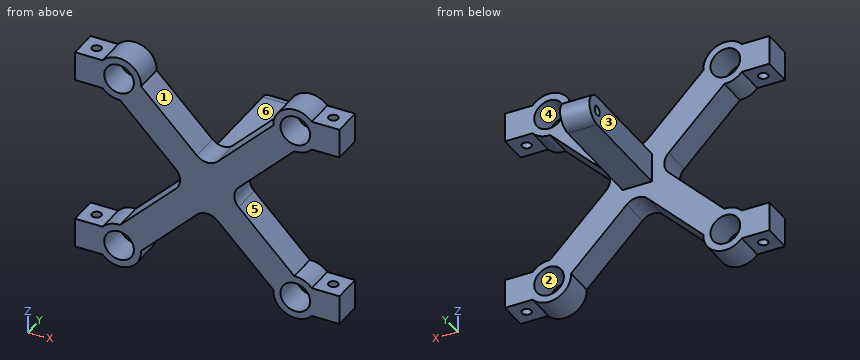
```python
from build123d import *

# Parameters (mm, degrees)
SKETCH_1_R          = 5.05
EXTRUDE_1_DEPTH     = 10
SKETCH_2_W          = 10
SKETCH_2_H          = 10
EXTRUDE_2_DEPTH     = 40
FILLET_3_RADIUS     = 5
FILLET_3_LENGTH     = 10
SKETCH_3_R          = 1.6
CUT_EXTRUDE_1_DEPTH = 81.039052968
SKETCH_4_R          = 1.6
CUT_EXTRUDE_2_DEPTH = 99.900202224


with BuildPart() as part:
    # ｽｹｯﾁ1 → ﾎﾞｽ - 押し出し1 (new body)
    with BuildSketch(Plane(origin=(0, 0, 0), x_dir=(1, 0, 0), z_dir=(0, 1, 0))):
        with BuildLine():
            Line((3.535533906, -10.677312396), (22.508173367, -29.649951857))
            ThreePointArc((22.508173367, -29.649951857), (27.161016322, -36.941914122), (35.590169944, -35))
            Line((35.590169944, -35), (45, -35))
            Line((45, -35), (45, -25))
            Line((45, -25), (35.590169944, -25))
            ThreePointArc((35.590169944, -25), (32.90120994, -23.08386084), (29.649951857, -22.508173367))
            Line((29.649951857, -22.508173367), (10.677312396, -3.535533906))
            ThreePointArc((10.677312396, -3.535533906), (9.212846302, 0), (10.677312396, 3.535533906))
            Line((10.677312396, 3.535533906), (29.649951857, 22.508173367))
            ThreePointArc((29.649951857, 22.508173367), (32.90120994, 23.08386084), (35.590169944, 25))
            Line((35.590169944, 25), (45, 25))
            Line((45, 25), (45, 35))
            Line((45, 35), (35.590169944, 35))
            ThreePointArc((35.590169944, 35), (27.161016322, 36.941914122), (22.508173367, 29.649951857))
            Line((22.508173367, 29.649951857), (3.535533906, 10.677312396))
            ThreePointArc((3.535533906, 10.677312396), (0, 9.212846302), (-3.535533906, 10.677312396))
            Line((-3.535533906, 10.677312396), (-22.508173367, 29.649951857))
            ThreePointArc((-22.508173367, 29.649951857), (-27.161016322, 36.941914122), (-35.590169944, 35))
            Line((-35.590169944, 35), (-45, 35))
            Line((-45, 35), (-45, 25))
            Line((-45, 25), (-35.590169944, 25))
            ThreePointArc((-35.590169944, 25), (-32.90120994, 23.08386084), (-29.649951857, 22.508173367))
            Line((-29.649951857, 22.508173367), (-10.677312396, 3.535533906))
            ThreePointArc((-10.677312396, 3.535533906), (-9.212846302, 0), (-10.677312396, -3.535533906))
            Line((-10.677312396, -3.535533906), (-29.649951857, -22.508173367))
            ThreePointArc((-29.649951857, -22.508173367), (-32.90120994, -23.08386084), (-35.590169944, -25))
            Line((-35.590169944, -25), (-45, -25))
            Line((-45, -25), (-45, -35))
            Line((-45, -35), (-35.590169944, -35))
            ThreePointArc((-35.590169944, -35), (-27.161016322, -36.941914122), (-22.508173367, -29.649951857))
            Line((-22.508173367, -29.649951857), (-3.535533906, -10.677312396))
            ThreePointArc((-3.535533906, -10.677312396), (0, -9.212846302), (3.535533906, -10.677312396))
        make_face()
        with Locations(Location((30, 30, 0), (0, 0, 270))):
            Circle(SKETCH_1_R, mode=Mode.SUBTRACT)
        with Locations(Location((-30, 30, 0), (0, 0, 90))):
            Circle(SKETCH_1_R, mode=Mode.SUBTRACT)
        with Locations(Location((30, -30, 0), (0, 0, 90))):
            Circle(SKETCH_1_R, mode=Mode.SUBTRACT)
        with Locations(Location((-30, -30, 0), (0, 0, 270))):
            Circle(SKETCH_1_R, mode=Mode.SUBTRACT)
    extrude(amount=EXTRUDE_1_DEPTH)

    # ｽｹｯﾁ2 → ﾎﾞｽ - 押し出し2 (add)
    with BuildSketch(Plane(origin=(0, 10, 0), x_dir=(1, 0, 0), z_dir=(0, 1, 0))):
        Rectangle(SKETCH_2_W, SKETCH_2_H)
    extrude(amount=EXTRUDE_2_DEPTH)

    # ﾌｨﾚｯﾄ3: full round fillet: the end face becomes a half cylinder, R = half its width
    fillet_3_face = Plane((0, 50, 0), x_dir=(-1, 0, 0), z_dir=(0, 1, 0))  # on the end face: x along it, z out of the body
    fillet_3_slab = fillet_3_face.offset(-FILLET_3_RADIUS / 2) * Box(FILLET_3_LENGTH, 2 * FILLET_3_RADIUS, FILLET_3_RADIUS, mode=Mode.PRIVATE)  # the body's end, R deep
    fillet_3_round = Plane((0, 45, 0), x_dir=(0, 1, 0), z_dir=(-1, 0, 0)) * Cylinder(FILLET_3_RADIUS, FILLET_3_LENGTH, mode=Mode.PRIVATE)  # its axis R under the face
    add(fillet_3_slab - fillet_3_round, mode=Mode.SUBTRACT)

    # ｽｹｯﾁ3 → ｶｯﾄ - 押し出し1 (cut, through all)
    with BuildSketch(Plane(origin=(5, 0, 0), x_dir=(0, 0, -1), z_dir=(1, 0, 0))):
        with Locations((0, 45)):
            Circle(SKETCH_3_R)
    extrude(amount=-CUT_EXTRUDE_1_DEPTH, mode=Mode.SUBTRACT)

    # ｽｹｯﾁ4 → ｶｯﾄ - 押し出し2 (cut, through all)
    with BuildSketch(Plane.XY.offset(35)):
        with Locations((-40.295084972, 5)):
            Circle(SKETCH_4_R)
        with Locations((40.295084972, 5)):
            Circle(SKETCH_4_R)
    extrude(amount=-CUT_EXTRUDE_2_DEPTH, mode=Mode.SUBTRACT)


solid = part.part
```
Check sheet for the modelled part. Datum: model origin and axes. Units: mm. Face numbers are marked on the shaded views. A direction names the side the tool comes from. Round coordinates to 2 decimals unless told otherwise and drop trailing zeros. Order: outer loops, then holes, each group sorted by start corner. A loop starts at its lowest first (then second) coordinate and runs counter-clockwise, first axis right, second up.
1) Section check D-D (z = 20). Record the boundary of the cut face in (x, y), and give its area (3 significant figures).
2) Tool access check on the marked faces 1 and 2. Record the directions out of +Z, -Z, +X, -X, +Y, -Y that give a thin tool (end or side, any length) a straight path to the whole face; none if there is none.
3) Section check B-B (y = 5). Give the number of separate pieces and of enclosed holes in the cut face, and give its area (3 significant figures).
4) Section check A-A (z = 0). Record the boundary of the cut face in (x, y).
5) Section check C-C (x = -21). Record the boundary of the cut face in (y, z), and give its area (3 significant figures).
6) Mould release check, pull along X, two halves, no side actions. Record for the marked faces 3, 4, 5 and 6: +X half, -X half, draft (parallel to the pull), parting line (faces both ways), or undercut.
7) Scan lines: line 1 (X direction, y = 2, z = 30); line 2 (Y direction, x = -2, z = 0); line 3 (Z direction, x = 33, y = 6.5). Record each from-to range of solid material in increasing order.
8) Go/stop test with flat-tipped pins: pin 1 Ø4.5 at (x, y) = (-42.5, 5.5) entering from -Z; pin 2 Ø10.5 at (x, y) = (39.5, 4.5) entering from -Z; pin 3 Ø16 at (x, z) = (30, 30) entering from +Y. Record where each tip stops, or that it passes through.
Result:
1. outline: (-27.14, 0) - (-12.86, 0) - (-12.86, 10) - (-27.14, 10) - close; (12.86, 0) - (27.14, 0) - (27.14, 10) - (12.86, 10) - close
1. area: 286 mm2
2. face 1: +Z, +Y, -Y
2. face 2: +Y, -Y
3. separate pieces: 5
3. enclosed holes: 4
3. area: 1,940 mm2
4. outline: (-9.21, 0) - (9.21, 0) - (9.21, 10) - (5, 10) - (5, 43.4) - (-5, 43.4) - (-5, 10) - (-9.21, 10) - close; (-5, 46.6) - (5, 46.6) - (5, 50) - (-5, 50) - close
5. outline: (0, -28.14) - (10, -28.14) - (10, -13.86) - (0, -13.86) - close; (0, 13.86) - (10, 13.86) - (10, 28.14) - (0, 28.14) - close
5. area: 286 mm2
6. face 3: -X half
6. face 4: undercut
6. face 5: +X half
6. face 6: draft
7. line 1: x = -45 to -35.05, -24.95 to -22.5, 22.5 to 24.95, 35.05 to 45
7. line 2: y = 0 to 43.4, 46.6 to 50
7. line 3: z = -36.87 to -34.06, -25.94 to -23.13, 23.13 to 25.94, 34.06 to 36.87
8. pin 1: stops at z = -35
8. pin 2: stops at z = -36.18
8. pin 3: stops at y = 10
